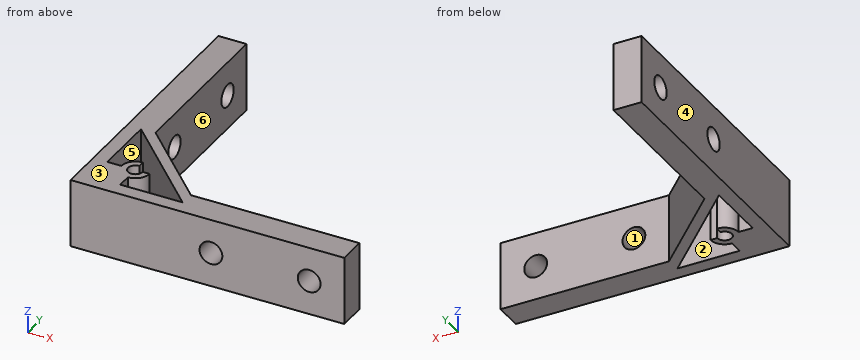
```python
from build123d import *

# Parameters (mm, degrees)
EXTRUDE_1_DEPTH     = 19.5
CUT_EXTRUDE_1_REACH = 114.019
EXTRUDE_2_DEPTH     = 19.5
CUT_EXTRUDE_2_REACH = 114.019
SKETCH_4_R          = 2.1
CUT_EXTRUDE_3_REACH = 108.603
SKETCH_5_R          = 3.25
CUT_EXTRUDE_4_REACH = 108.603
SKETCH_6_R          = 3.25


with BuildPart() as part:
    # 草图1 → 凸台-拉伸1 (new body)
    with BuildSketch(Plane.XY):
        Polygon((0, 0), (78, 0), (78, 8), (30, 8), (8, 30), (8, 78), (0, 78), align=None)
    extrude(amount=EXTRUDE_1_DEPTH)

    # 草图2 → 切除-拉伸1 (cut, up to next)
    with BuildSketch(Plane.XY.offset(19.5), mode=Mode.PRIVATE) as cut_extrude_1_sk1:
        Polygon((4, 29.757359313), (29.757359313, 4), (12, 4), (12, 12), (4, 12), align=None)
    cut_extrude_1_tool1 = extrude(cut_extrude_1_sk1.sketch, amount=-CUT_EXTRUDE_1_REACH, mode=Mode.PRIVATE) & part.part
    add(cut_extrude_1_tool1.solids().sort_by_distance((13.682042, 13.682042, 19.5))[0], mode=Mode.SUBTRACT)

    # 草图3 → 凸台-拉伸2 (add)
    with BuildSketch(Plane.XY.offset(19.5)):
        with BuildLine():
            Line((12, 12), (12, 16))
            ThreePointArc((12, 16), (9.171572875, 9.171572875), (16, 12))
            Line((16, 12), (12, 12))
        make_face()
    extrude(amount=-EXTRUDE_2_DEPTH)

    # 草图4 → 切除-拉伸2 (cut, up to next)
    with BuildSketch(Plane.XY.offset(19.5), mode=Mode.PRIVATE) as cut_extrude_2_sk1:
        with Locations((12, 12)):
            Circle(SKETCH_4_R)
    cut_extrude_2_tool1 = extrude(cut_extrude_2_sk1.sketch, amount=-CUT_EXTRUDE_2_REACH, mode=Mode.PRIVATE) & part.part
    add(cut_extrude_2_tool1.solids().sort_by_distance((12, 12, 19.5))[0], mode=Mode.SUBTRACT)

    # 草图5 → 切除-拉伸3 (cut, up to next)
    with BuildSketch(Plane(origin=(0, 8, 0), x_dir=(1, 0, 0), z_dir=(0, 1, 0)), mode=Mode.PRIVATE) as cut_extrude_3_sk1:
        with Locations(Location((40, -9.75, 0), (0, 0, 180))):
            Circle(SKETCH_5_R)
    cut_extrude_3_tool1 = extrude(cut_extrude_3_sk1.sketch, amount=-CUT_EXTRUDE_3_REACH, mode=Mode.PRIVATE) & part.part
    # 草图5 → 切除-拉伸3 (cut, up to next)
    with BuildSketch(Plane(origin=(0, 8, 0), x_dir=(1, 0, 0), z_dir=(0, 1, 0)), mode=Mode.PRIVATE) as cut_extrude_3_sk2:
        with Locations(Location((68, -9.75, 0), (0, 0, 180))):
            Circle(SKETCH_5_R)
    cut_extrude_3_tool2 = extrude(cut_extrude_3_sk2.sketch, amount=-CUT_EXTRUDE_3_REACH, mode=Mode.PRIVATE) & part.part
    add(cut_extrude_3_tool1.solids().sort_by_distance((40, 8, 9.75))[0], mode=Mode.SUBTRACT)
    add(cut_extrude_3_tool2.solids().sort_by_distance((68, 8, 9.75))[0], mode=Mode.SUBTRACT)

    # 草图6 → 切除-拉伸4 (cut, up to next)
    with BuildSketch(Plane(origin=(8, 0, 0), x_dir=(0, 0, -1), z_dir=(1, 0, 0)), mode=Mode.PRIVATE) as cut_extrude_4_sk1:
        with Locations((-9.75, 68)):
            Circle(SKETCH_6_R)
    cut_extrude_4_tool1 = extrude(cut_extrude_4_sk1.sketch, amount=-CUT_EXTRUDE_4_REACH, mode=Mode.PRIVATE) & part.part
    # 草图6 → 切除-拉伸4 (cut, up to next)
    with BuildSketch(Plane(origin=(8, 0, 0), x_dir=(0, 0, -1), z_dir=(1, 0, 0)), mode=Mode.PRIVATE) as cut_extrude_4_sk2:
        with Locations((-9.75, 40)):
            Circle(SKETCH_6_R)
    cut_extrude_4_tool2 = extrude(cut_extrude_4_sk2.sketch, amount=-CUT_EXTRUDE_4_REACH, mode=Mode.PRIVATE) & part.part
    add(cut_extrude_4_tool1.solids().sort_by_distance((8, 68, 9.75))[0], mode=Mode.SUBTRACT)
    add(cut_extrude_4_tool2.solids().sort_by_distance((8, 40, 9.75))[0], mode=Mode.SUBTRACT)


solid = part.part
```
Verification items for the finished model (mm, model axes). Face numbers are marked on the shaded views. A direction names the side the tool comes from. Give positions to 0.01 mm unless a question says otherwise; leave off trailing zeros. Order: outer loops, then holes, each group sorted by start corner. A loop starts at its lowest first (then second) coordinate and runs counter-clockwise, first axis right, second up. Notation, with made-up numbers: M -22,-35 L 26,-35 A33 ccw 26,2 Z; hole C 7,18.5 d11. An arc over 180 degrees is marked long. Answer in a Markdown table with one row per item. Add a question column.
Item 1: Mould release check, pull along Z, two halves, no side actions. Record for the marked faces 1, 2 and 3: released by +Z, released by -Z, zero draft, split by the parting line, or undercut.
Item 2: Section check B-B, the plane z = 9.75. State how many separate pieces and enclosed holes the cut face has, and give its area (3 significant figures).
Item 3: Scan lines: probe 1 along Y at (x, z) = (2, 9.75); probe 2 along Z at (x, y) = (40, 4.25); probe 3 along Y at (x, z) = (14.5, 16.5). Record each from-to range of solid material in increasing order. Write a range as from..to.
Item 4: Section check A-A, the plane x = 68. Enter the section's corners in (y, z).
Item 5: Tool access check on the marked faces 4, 5 and 6. Record the directions out of +Z, -Z, +X, -X, +Y, -Y that give a thin tool (end or side, any length) a straight path to the whole face; none if there is none.
Item 6: Section check D-D, the plane z = 15. Enter the section's corners in (x, y).
Item 7: Gauge pin test, flat ends, axial feed: pin 1 (7.5 mm diameter, centred on y = 68, z = 9.75, fed in from +X); pin 2 (1.5 mm diameter, centred on y = 15, z = 10, fed in from +X); pin 3 (4 mm diameter, centred on x = 13.5, z = 4, fed in from -Y); pin 4 (5 mm diameter, centred on x = 68, z = 9.75, fed in from -Y). Record the tip position at first contact, or that the pin passes through.
Filled sheet:
| question | item | result |
|---|---|---|
| 1 | face 1 | undercut |
| 1 | face 2 | zero draft |
| 1 | face 3 | released by +Z |
| 2 | separate pieces | 5 |
| 2 | enclosed holes | 1 |
| 2 | area | 965 mm^2 |
| 3 | probe 1 | y = 0..36.75, 43.25..64.75, 71.25..78 |
| 3 | probe 2 | z = 0..6.5, 13..19.5 |
| 3 | probe 3 | y = 0..4, 8.88..12, 19.26..23.5 |
| 4 | outline | M 0,0 L 8,0 L 8,6.5 L 0,6.5 Z; M 0,13 L 8,13 L 8,19.5 L 0,19.5 Z |
| 5 | face 4 | +Z, -Z, -X, +Y, -Y |
| 5 | face 5 | +Z, -Z |
| 5 | face 6 | +Z, -Z, +X, +Y |
| 6 | outline | M 0,0 L 78,0 L 78,8 L 30,8 L 8,30 L 8,78 L 0,78 Z; hole M 4,12 L 8,12 A4 cw 12,16 L 12,14.1 A2.1 ccw long 14.1,12 L 16,12 A4 cw 12,8 L 12,4 L 29.76,4 L 4,29.76 Z |
| 7 | pin 1 | stops at x = 8 |
| 7 | pin 2 | stops at x = 23.75 |
| 7 | pin 3 | stops at y = 0 |
| 7 | pin 4 | passes through |
